Geometry check sheet. Reference: the model listing, model coordinates, mm. A direction names the side the tool comes from. Give positions to 0.01 mm unless a question says otherwise; leave off trailing zeros. Use a Markdown table: item, result. Add a question column.
1. Draft check along Z on faces 1 (the flat face through (538, 110, 10)), 2 (the cylindrical face through (277.3, 34.96, 1.43)), 3 (the cylindrical face through (810.12, 33.52, 48.57)). Enter one of: pulls with the +Z half, pulls with the -Z half, needs draft (parallel to the pull), parting line crosses it, or undercut.
2. Depth check by flat-ended pin: P1, Ø10, axis at x = 126.5, z = 19.5, coming from the -Y side; P2, Ø5, axis at y = 0, z = 20.5, coming from the -X side; P3, Ø10, axis at x = 614.5, z = 33.5, coming from the -Y side; P4, Ø8, axis at x = 740, y = 81, coming from the -Z side. Enter the tip coordinate at first touch or a pass-through.
3. Material ranges on L1, parallel to Z at x = 417, y = 105; L2, parallel to Y at x = 537, z = 29; L3, parallel to Y at x = 592.5, z = 41, recorded low to high.
4. Set-up check for faces 4 (the flat face through (14.1, 32.43, 24.72)), 5 (the cylindrical face through (796.669, 78.79, 1.504)), 6 (the cylindrical face through (810.12, 33.52, 1.43)): record each of +Z, -Z, +X, -X, +Y, -Y from which the full face is reachable in a straight line by a thin tool's end or side.
from build123d import *

# Parameters (mm, degrees)
DODANIE_WYCI_GNI_CIE1_DEPTH = 50
DODANIE_WYCI_GNI_CIE4_DEPTH = 10
DODANIE_WYCI_GNI_CIE5_DEPTH = 10
ZAOKR_GLENIE1_R             = 5


with BuildPart() as part:
    # Szkic1 → Dodanie-wyciągnięcie1 (new body)
    with BuildSketch(Plane.XY):
        Polygon((1060.363636364, 3.796475094), (540, 104.403065089), (19.636363636, 3.796475094), (10.145175901, 52.887384185), (-9.491187735, 49.090909091), (0, 0), (3.796475094, -19.636363636), (540, 84.403065089), (1076.203524906, -19.636363636), (1080, 0), (1089.491187735, 49.090909091), (1069.854824099, 52.887384185), align=None)
    extrude(amount=DODANIE_WYCI_GNI_CIE1_DEPTH)

    # Szkic4 → Dodanie-wyciągnięcie4 (add)
    with BuildSketch(Plane.XY.offset(50)):
        Polygon((19.636363636, 3.796475094), (14.890769769, 28.34192964), (540, 129.866028052), (1065.109230231, 28.34192964), (1060.363636364, 3.796475094), (540, 104.403065089), align=None)
    extrude(amount=-DODANIE_WYCI_GNI_CIE4_DEPTH)

    # Szkic5 → Dodanie-wyciągnięcie5 (add)
    with BuildSketch(Plane(origin=(0, 0, 0), x_dir=(-1, 0, 0), z_dir=(0, 0, -1))):
        Polygon((-1060.363636364, 3.796475094), (-1065.109230231, 28.34192964), (-540, 129.866028052), (-14.890769769, 28.34192964), (-19.636363636, 3.796475094), (-540, 104.403065089), align=None)
    extrude(amount=-DODANIE_WYCI_GNI_CIE5_DEPTH)

    # Zaokrąglenie1
    zaokr_glenie1_edges = [part.edges().sort_by_distance(p)[0] for p in [
        (271.898237547, 32.383350726, 50),
        (1082.847356321, 14.727272727, 0),
        (1079.673005917, 50.989146638, 0),
        (1067.482027165, 40.614656912, 0),
        (12.517972835, 40.614656912, 0),
        (-2.847356321, 14.727272727, 50),
        (0.326994083, 50.989146638, 0),
        (-2.847356321, 14.727272727, 0),
        (271.898237547, 32.383350726, 0),
        (808.101762453, 32.383350726, 0),
        (0.326994083, 50.989146638, 50),
        (1089.491187735, 49.090909091, 25),
        (1069.854824099, 52.887384185, 25),
        (10.145175901, 52.887384185, 25),
        (-9.491187735, 49.090909091, 25),
        (3.796475094, -19.636363636, 25),
        (540, 84.403065089, 25),
        (1076.203524906, -19.636363636, 25),
        (12.517972835, 40.614656912, 50),
        (1067.482027165, 40.614656912, 50),
        (1079.673005917, 50.989146638, 50),
        (19.636363636, 3.796475094, 25),
        (540, 104.403065089, 25),
        (1060.363636364, 3.796475094, 25),
        (279.818181818, 54.099770092, 40),
        (17.263566703, 16.069202367, 40),
        (1082.847356321, 14.727272727, 50),
        (277.445384884, 79.103978846, 40),
        (14.890769769, 28.34192964, 45),
        (802.554615116, 79.103978846, 40),
        (540, 129.866028052, 45),
        (1062.736433297, 16.069202367, 40),
        (1065.109230231, 28.34192964, 45),
        (800.181818182, 54.099770092, 40),
        (802.554615116, 79.103978846, 50),
        (277.445384884, 79.103978846, 50),
        (800.181818182, 54.099770092, 10),
        (1062.736433297, 16.069202367, 10),
        (802.554615116, 79.103978846, 10),
        (1065.109230231, 28.34192964, 5),
        (277.445384884, 79.103978846, 10),
        (540, 129.866028052, 5),
        (17.263566703, 16.069202367, 10),
        (14.890769769, 28.34192964, 5),
        (279.818181818, 54.099770092, 10),
        (277.445384884, 79.103978846, 0),
        (802.554615116, 79.103978846, 0),
        (808.101762453, 32.383350726, 50),
    ]]
    fillet(zaokr_glenie1_edges, radius=ZAOKR_GLENIE1_R - 0.0001)  # a hair under: the kernel refuses the full size


solid = part.part
Values found:
| question | item | result |
|---|---|---|
| 1 | face 1 | undercut |
| 1 | face 2 | pulls with the -Z half |
| 1 | face 3 | pulls with the +Z half |
| 2 | P1 | stops at y = 3.2 |
| 2 | P2 | stops at x = -0.48 |
| 2 | P3 | stops at y = 68.98 |
| 2 | P4 | stops at z = 0 |
| 3 | L1 | z = 1.91 to 8.09, 41.91 to 48.09 |
| 3 | L2 | y = 83.82 to 103.82 |
| 3 | L3 | y = 74.22 to 117.68 |
| 4 | face 4 | +Y |
| 4 | face 5 | -Z, +Y |
| 4 | face 6 | -Z, -Y |
